The model under review builds one solid part; all positions refer to its coordinate system, in mm. A direction names the side the tool comes from. Round coordinates to 2 decimals unless told otherwise and drop trailing zeros. Order: outer loops, then holes, each group sorted by start corner. A loop starts at its lowest first (then second) coordinate and runs counter-clockwise, first axis right, second up. Notation, with made-up numbers: M -21.5,13.5 L 0.5,13.5 A24 ccw 0.5,50.5 Z; hole C 75,27 d5. An arc over 180 degrees is marked long. Answer as a JSON object with one key per item and string values. Group by question number.
1. Add section C-C on z = 74.5. State the section outline as (x, y) points.
2. Add section D-D on x = 20. State the section outline as (y, z) points.
3. Mouldability with a two-part tool opening along Y and no side actions: class faces 1 (the face through (-2, -150, 59)), 2 (the face through (112, 2, 118)), 3 (the face through (-130, -2, 59)) as released by +Y, released by -Y, zero draft, split by the parting line, or undercut.
4. Add section A-A on y = -127. State the section outline as (x, z) points.
5. To check wall thickness, follow probe 1 along Y at (x, z) = (-81, 13); probe 2 along Y at (x, z) = (-6.5, 22.5); probe 3 along X at (y, z) = (-91, 26). State the ranges of each line that lie inside material, in increasing order. Write a range as [from, to].
6. Machinability: for faces 4 (the face through (130, -2, 59)), 5 (the face through (-2, 2, 2)), which of the approach directions +Z, -Z, +X, -X, +Y, -Y give a long, thin tool a straight path to every point of the face, cutting with its end or side? Answer none if there is none.
7. Clearance check with flat-ended pins moving along their axes: P1, Ø2.5, axis at x = -36, y = -87, coming from the +Z side; P2, Ø6, axis at x = -50.5, y = 115, coming from the +Z side; P3, Ø5, axis at x = 54.5, y = -19.5, coming from the -Z side. State where each tip first meets the part, or that it passes through.
8. Add section B-B on x = 104. State the section outline as (y, z) points, and give its area (3 significant figures).
```python
from build123d import *

# Parameters (mm, degrees)
CROQUIS2_W              = 260
CROQUIS2_H              = 300
SALIENTE_EXTRUIR1_DEPTH = 120
CROQUIS3_W              = 200
CROQUIS3_H              = 240
CORTAR_EXTRUIR2_DEPTH   = 2
CROQUIS4_W              = 256
CROQUIS4_H              = 296
CORTAR_EXTRUIR3_DEPTH   = 116
CROQUIS6_W              = 117
CROQUIS6_H              = 3
SALIENTE_EXTRUIR2_DEPTH = 120


with BuildPart() as part:
    # Croquis2 → Saliente-Extruir1 (new body)
    with BuildSketch(Plane.XY):
        Rectangle(CROQUIS2_W, CROQUIS2_H)
    extrude(amount=SALIENTE_EXTRUIR1_DEPTH)

    # Croquis3 → Cortar-Extruir2 (cut)
    with BuildSketch(Plane.XY.offset(120)):
        Rectangle(CROQUIS3_W, CROQUIS3_H)
    extrude(amount=-CORTAR_EXTRUIR2_DEPTH, mode=Mode.SUBTRACT)

    # Croquis4 → Cortar-Extruir3 (cut)
    with BuildSketch(Plane.XY.offset(118)):
        Rectangle(CROQUIS4_W, CROQUIS4_H)
    extrude(amount=-CORTAR_EXTRUIR3_DEPTH, mode=Mode.SUBTRACT)

    # Croquis6 → Saliente-Extruir2 (add)
    with BuildSketch(Plane(origin=(-128, 0, 0), x_dir=(0, 0, -1), z_dir=(1, 0, 0))):
        with Locations((-60.5, -86.5)):
            Rectangle(CROQUIS6_W, CROQUIS6_H)
    extrude(amount=SALIENTE_EXTRUIR2_DEPTH)


solid = part.part
```
Recorded:
{
 "1": {"outline": "M -130,-150 L 130,-150 L 130,150 L -130,150 Z; hole M -128,-148 L 128,-148 L 128,148 L -128,148 L -128,-85 L -8,-85 L -8,-88 L -128,-88 Z"},
 "2": {"outline": "M -150,0 L 150,0 L 150,120 L 120,120 L 120,118 L 148,118 L 148,2 L -148,2 L -148,118 L -120,118 L -120,120 L -150,120 Z"},
 "3": {"face 1": "released by -Y", "face 2": "undercut", "face 3": "zero draft"},
 "4": {"outline": "M -130,0 L 130,0 L 130,120 L -130,120 Z; hole M -128,2 L 128,2 L 128,118 L -128,118 Z"},
 "5": {"probe 1": "y = [-150, -148], [-88, -85], [148, 150]", "probe 2": "y = [-150, -148], [148, 150]", "probe 3": "x = [-130, -128], [128, 130]"},
 "6": {"face 4": "+Z, -Z, +X, +Y, -Y", "face 5": "none"},
 "7": {"P1": "stops at z = 119", "P2": "stops at z = 2", "P3": "stops at z = 0"},
 "8": {"outline": "M -150,0 L 150,0 L 150,120 L -150,120 Z; hole M -148,2 L 148,2 L 148,118 L -148,118 Z", "area": "1,660 mm²"}
}
